For this review, take the finished solid that the model builds, in its own axes (mm). Face numbers are marked on the shaded views. A direction names the side the tool comes from. Round coordinates to 2 decimals unless told otherwise and drop trailing zeros. Order: outer loops, then holes, each group sorted by start corner. A loop starts at its lowest first (then second) coordinate and runs counter-clockwise, first axis right, second up. Notation, with made-up numbers: M 78,78 L 85,78 A14 ccw 85,104 Z; hole C 73.25,5.5 d1. An arc over 180 degrees is marked long. Put each result on its own line as item: value.
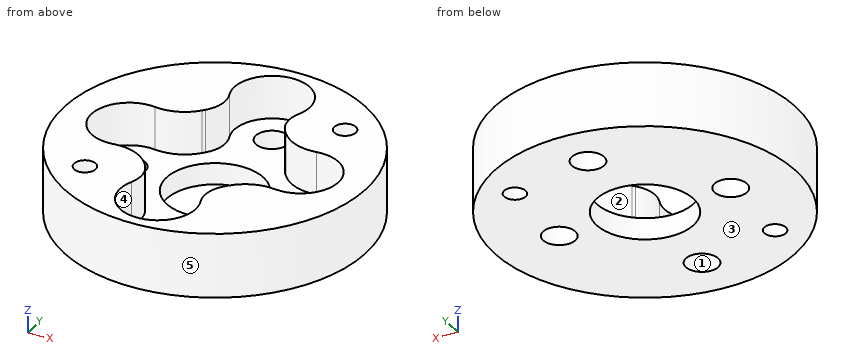
from build123d import *

# Parameters (mm, degrees)
SKETCH_1_R          = 14
EXTRUDE_1_DEPTH     = 2
SKETCH_2_R          = 1.5
SKETCH_2_R_2        = 4.5
CUT_EXTRUDE_1_DEPTH = 3
SKETCH_3_R          = 14
SKETCH_3_R_2        = 1
EXTRUDE_3_DEPTH     = 4
SKETCH_4_R          = 1
CUT_EXTRUDE_2_DEPTH = 7


with BuildPart() as part:
    # 草图1 → 凸台-拉伸1 (new body)
    with BuildSketch(Plane.XY):
        Circle(SKETCH_1_R)
    extrude(amount=EXTRUDE_1_DEPTH)

    # 草图2 → 切除-拉伸1 (cut, through all)
    with BuildSketch(Plane.XY.offset(2)):
        with Locations((-8, 0)):
            Circle(SKETCH_2_R)
        with Locations((0, 9.5)):
            Circle(SKETCH_2_R)
        with Locations((8, 0)):
            Circle(SKETCH_2_R)
        with Locations((0, -9.5)):
            Circle(SKETCH_2_R)
        Circle(SKETCH_2_R_2)
    extrude(amount=-CUT_EXTRUDE_1_DEPTH, mode=Mode.SUBTRACT)

    # 草图3 → 凸台-拉伸3 (add)
    with BuildSketch(Plane.XY.offset(2)):
        Circle(SKETCH_3_R)
        with Locations((-7.778174593, -7.778174593)):
            Circle(SKETCH_3_R_2, mode=Mode.SUBTRACT)
        with Locations((7.778174593, 7.778174593)):
            Circle(SKETCH_3_R_2, mode=Mode.SUBTRACT)
        with BuildLine():
            Line((-3.913416822, -4.852817524), (-3.714267904, -5.089306864))
            ThreePointArc((-3.714267904, -5.089306864), (-3.044670654, -6.56047377), (-3.235616191, -8.165538362))
            ThreePointArc((-3.235616191, -8.165538362), (0, -13), (3.235616191, -8.165538362))
            ThreePointArc((3.235616191, -8.165538362), (3.044670654, -6.56047377), (3.714267904, -5.089306864))
            Line((3.714267904, -5.089306864), (3.913416822, -4.852817524))
            ThreePointArc((3.913416822, -4.852817524), (5.538640325, -3.695403416), (7.520762087, -3.467034904))
            ThreePointArc((7.520762087, -3.467034904), (11.5, 0), (7.520762087, 3.467034904))
            ThreePointArc((7.520762087, 3.467034904), (5.538640325, 3.695403416), (3.913416822, 4.852817524))
            Line((3.913416822, 4.852817524), (3.714267904, 5.089306864))
            ThreePointArc((3.714267904, 5.089306864), (3.044670654, 6.56047377), (3.235616191, 8.165538362))
            ThreePointArc((3.235616191, 8.165538362), (0, 13), (-3.235616191, 8.165538362))
            ThreePointArc((-3.235616191, 8.165538362), (-3.044670654, 6.56047377), (-3.714267904, 5.089306864))
            Line((-3.714267904, 5.089306864), (-3.913416822, 4.852817524))
            ThreePointArc((-3.913416822, 4.852817524), (-5.538640325, 3.695403416), (-7.520762087, 3.467034904))
            ThreePointArc((-7.520762087, 3.467034904), (-11.5, 0), (-7.520762087, -3.467034904))
            ThreePointArc((-7.520762087, -3.467034904), (-5.538640325, -3.695403416), (-3.913416822, -4.852817524))
        make_face(mode=Mode.SUBTRACT)
    extrude(amount=EXTRUDE_3_DEPTH)

    # 草图4 → 切除-拉伸2 (cut, through all)
    with BuildSketch(Plane.XY.offset(6)):
        with Locations((7.778174593, 7.778174593)):
            Circle(SKETCH_4_R)
        with Locations((-7.778174593, -7.778174593)):
            Circle(SKETCH_4_R)
    extrude(amount=-CUT_EXTRUDE_2_DEPTH, mode=Mode.SUBTRACT)


solid = part.part
(1) Insertion check: pin 1 Ø4 at (x, y) = (0, -9.5) entering from -Z; pin 2 Ø2 at (x, z) = (-5.5, 5) entering from +Y; pin 3 Ø1 at (y, z) = (4.5, 5.5) entering from -X; pin 4 Ø2 at (x, z) = (-2.5, 4) entering from +Y. Each pin has a flat end and moves straight along its axis. Give the tip position at first contact, or say it passes through.
A:
pin 1: stops at z = 0
pin 2: stops at y = 13.26
pin 3: stops at x = -13.42
pin 4: stops at y = 13.92
(2) Draft analysis for pull direction X (two halves, no side actions). For the marked faces 3, 4 and 5, state which applies: released by +X, released by -X, zero draft, split by the parting line, or undercut.
A:
face 3: zero draft
face 4: undercut
face 5: split by the parting line
(3) For the marked faces 1 and 2, list the 3-axis set-ups (+Z, -Z, +X, -X, +Y, -Y) from which the entire face can be reached by the end or side of a thin tool; tool diameter is ignored.
A:
face 1: +Z, -Z
face 2: +Z
(4) To check wall thickness, follow L1, parallel to Y at x = 0, z = 0.75; L2, parallel to Y at x = 0, z = 3.3; L3, parallel to X at y = 7.25, z = 5.25. State the ranges of each line that lie inside material, in increasing order.
A:
L1: y = -14 to -11, -8 to -4.5, 4.5 to 8, 11 to 14
L2: y = -14 to -13, 13 to 14
L3: x = -11.98 to -3.02, 3.02 to 6.93, 8.63 to 11.98
(5) Add section A-A on x = 0. Give the boundary of the cut face in (y, z), then the cut area to 3 significant figures.
A:
outline: M -14,0 L -11,0 L -11,2 L -13,2 L -13,6 L -14,6 Z; M -8,0 L -4.5,0 L -4.5,2 L -8,2 Z; M 4.5,0 L 8,0 L 8,2 L 4.5,2 Z; M 11,0 L 14,0 L 14,6 L 13,6 L 13,2 L 11,2 Z
area: 34.0 mm2
(6) Add section D-D on z = 0.85. Give the boundary of the cut face in (x, y).
A:
outline: C 0,0 d28; hole C -8,0 d3; hole C -7.78,-7.78 d2; hole C 0,0 d9; hole C 0,-9.5 d3; hole C 0,9.5 d3; hole C 8,0 d3; hole C 7.78,7.78 d2
(7) Add section C-C on x = -8. Give the boundary of the cut face in (y, z), then the cut area to 3 significant figures.
A:
outline: M -11.49,0 L -8.75,0 L -8.75,6 L -11.49,6 Z; M -6.8,0 L -1.5,0 L -1.5,2 L -3.5,2 L -3.5,6 L -6.8,6 Z; M 1.5,0 L 11.49,0 L 11.49,6 L 3.5,6 L 3.5,2 L 1.5,2 Z
area: 92.2 mm2
(8) Add section B-B on y = 0. Give the boundary of the cut face in (x, z), then the cut area to 3 significant figures.
A:
outline: M -14,0 L -9.5,0 L -9.5,2 L -11.5,2 L -11.5,6 L -14,6 Z; M -6.5,0 L -4.5,0 L -4.5,2 L -6.5,2 Z; M 4.5,0 L 6.5,0 L 6.5,2 L 4.5,2 Z; M 9.5,0 L 14,0 L 14,6 L 11.5,6 L 11.5,2 L 9.5,2 Z
area: 46.0 mm2
